```python
from build123d import *

# Parameters (mm, degrees)
BOSS_EXTRUDE7_DEPTH                          = 17
BOSS_EXTRUDE7_DEPTH_BACK                     = 17
SKETCH1_R                                    = 1.45
SKETCH34_W                                   = 28.4
SKETCH34_H                                   = 7.5
CUT_EXTRUDE11_DEPTH                          = 37.521397837
SKETCH35_R                                   = 5
CUT_EXTRUDE12_DEPTH                          = 25.542055741
CSK_FOR_M3_HEX_SOCKET_COUNTERSUNK_CA_2_COUNT = 2
CSK_FOR_M3_HEX_SOCKET_COUNTERSUNK_CA_2_PITCH = 16.5
CSK_FOR_M3_HEX_SOCKET_COUNTERSUNK_CA_3_COUNT = 2
CSK_FOR_M3_HEX_SOCKET_COUNTERSUNK_CA_3_PITCH = 18
CSK_FOR_M3_HEX_SOCKET_COUNTERSUNK_CA_4_COUNT = 2
CSK_FOR_M3_HEX_SOCKET_COUNTERSUNK_CA_4_PITCH = 24.418230894
FILLET5_R                                    = 1
SKETCH41_W                                   = 28.5
SKETCH41_H                                   = 0.4
CUT_EXTRUDE13_DEPTH                          = 40.895175147


with BuildPart() as part:
    # Sketch1 → Boss-Extrude7 (new, two sides: drawn at the far end of the back side and taken through both)
    # profile 1 of 3: a face of its own
    with BuildSketch(Plane.XY.offset(-BOSS_EXTRUDE7_DEPTH_BACK)):
        Polygon((-14.25, 15.25), (-14.25, 11.25), (-8.25, 11.25), (-8.25, 12.25), (8.25, 12.25), (8.25, 11.25), (14.25, 11.25), (14.25, 15.25), align=None)
    # profile 2 of 3: a face of its own
    with BuildSketch(Plane.XY.offset(-BOSS_EXTRUDE7_DEPTH_BACK)):
        with BuildLine():
            Line((14.25, 4.75), (14.25, 11.25))
            Line((14.25, 11.25), (8.25, 11.25))
            Line((8.25, 11.25), (8.25, 8.011710179))
            ThreePointArc((8.25, 8.011710179), (9.502581542, 6.476954843), (10.473180033, 4.75))
            Line((10.473180033, 4.75), (14.25, 4.75))
        make_face()
        with Locations((11, 8)):
            Circle(SKETCH1_R, mode=Mode.SUBTRACT)
    # profile 3 of 3: a face of its own
    with BuildSketch(Plane.XY.offset(-BOSS_EXTRUDE7_DEPTH_BACK)):
        with BuildLine():
            Line((-8.25, 11.25), (-14.25, 11.25))
            Line((-14.25, 11.25), (-14.25, 4.75))
            Line((-14.25, 4.75), (-10.473180033, 4.75))
            ThreePointArc((-10.473180033, 4.75), (-9.502581542, 6.476954843), (-8.25, 8.011710179))
            Line((-8.25, 8.011710179), (-8.25, 11.25))
        make_face()
        with Locations((-11, 8)):
            Circle(SKETCH1_R, mode=Mode.SUBTRACT)
    extrude(amount=BOSS_EXTRUDE7_DEPTH + BOSS_EXTRUDE7_DEPTH_BACK)

    # Sketch34 → Cut-Extrude11 (cut, through all)
    with BuildSketch(Plane.ZY.offset(14.25)):
        with Locations((0, 8.5)):
            Rectangle(SKETCH34_W, SKETCH34_H)
    extrude(amount=-CUT_EXTRUDE11_DEPTH, mode=Mode.SUBTRACT)

    # Sketch35 → Cut-Extrude12 (cut, through all)
    with BuildSketch(Plane(origin=(0, 15.25, 0), x_dir=(1, 0, 0), z_dir=(0, 1, 0))):
        with Locations(Location((0, 0, 0), (0, 0, 270))):
            Circle(SKETCH35_R)
    extrude(amount=-CUT_EXTRUDE12_DEPTH, mode=Mode.SUBTRACT)

    # Sketch40 → CSK for M3 Hex Socket Countersunk Cap Sc (revolve, cut)
    with BuildSketch(Plane(origin=(-8.25, 12.25, 9), x_dir=(0, 0, -1), z_dir=(1, 0, 0))):
        Polygon((0, 0), (0, 3), (1.7, 3), (1.7, 1.66), (3.36, 0), align=None)
    csk_for_m3_hex_socket_countersunk_cap_sc = revolve(axis=Axis((-8.25, 5.9, 9), (0, 1, 0)), mode=Mode.SUBTRACT)

    # CSK for M3 Hex Socket Countersunk Ca 2: CSK for M3 Hex Socket Countersunk Cap Sc ×2
    with Locations(*[(i * CSK_FOR_M3_HEX_SOCKET_COUNTERSUNK_CA_2_PITCH, 0, 0) for i in range(1, CSK_FOR_M3_HEX_SOCKET_COUNTERSUNK_CA_2_COUNT)]):
        add(csk_for_m3_hex_socket_countersunk_cap_sc, mode=Mode.SUBTRACT)

    # CSK for M3 Hex Socket Countersunk Ca 3: CSK for M3 Hex Socket Countersunk Cap Sc ×2
    with Locations(*[(0, 0, -i * CSK_FOR_M3_HEX_SOCKET_COUNTERSUNK_CA_3_PITCH) for i in range(1, CSK_FOR_M3_HEX_SOCKET_COUNTERSUNK_CA_3_COUNT)]):
        add(csk_for_m3_hex_socket_countersunk_cap_sc, mode=Mode.SUBTRACT)

    # CSK for M3 Hex Socket Countersunk Ca 4: CSK for M3 Hex Socket Countersunk Cap Sc ×2
    with Locations(*[Vector(0.6757246285173466, 0, -0.7371541402007413) * (i * CSK_FOR_M3_HEX_SOCKET_COUNTERSUNK_CA_4_PITCH) for i in range(1, CSK_FOR_M3_HEX_SOCKET_COUNTERSUNK_CA_4_COUNT)]):
        add(csk_for_m3_hex_socket_countersunk_cap_sc, mode=Mode.SUBTRACT)

    # Fillet5
    fillet5_edges = [part.edges().sort_by_distance(p)[0] for p in [
        (-14.25, 15.25, 0),
        (14.25, 15.25, 0),
        (0, 15.25, -17),
        (0, 15.25, 17),
    ]]
    fillet(fillet5_edges, radius=FILLET5_R)

    # Sketch41 → Cut-Extrude13 (cut, through all)
    with BuildSketch(Plane.XY.offset(17)):
        with Locations((0, 4.95)):
            Rectangle(SKETCH41_W, SKETCH41_H)
    extrude(amount=-CUT_EXTRUDE13_DEPTH, mode=Mode.SUBTRACT)


solid = part.part
```
Geometry check sheet. Reference: the model listing, model coordinates, mm. A direction names the side the tool comes from. Coordinates: 2 decimals unless noted, no trailing zeros. Order: outer loops, then holes, each group sorted by start corner. A loop starts at its lowest first (then second) coordinate and runs counter-clockwise, first axis right, second up. Notation, with made-up numbers: (11, 78) - (36, 78) arc R20 cw to (36, 92) - close; hole circle Ø1 at (1.25, -8). An arc over 180 degrees is marked (long way). Answer as a JSON object with one key per item and string values. Group by question number.
Item 1: Sectioned sample at A-A, the plane z = -9. Record the cut outline in (x, y), and give its area (3 significant figures).
Item 2: Depth check by flat-ended pin: pin 1 Ø1.8 at (x, y) = (-11.5, 9) entering from -Z. Enter the tip coordinate at first touch or a pass-through.
Item 3: Sectioned sample at B-B, the plane y = 10.5. Record the cut outline in (x, z).
Item 4: Sectioned sample at D-D, the plane x = -12. Record the cut outline in (y, z), and give its area (3 significant figures).
Item 5: Scan lines: probe 1 along X at (y, z) = (14.55, 9); probe 2 along Z at (x, y) = (12.25, 9.5); probe 3 along Z at (x, y) = (-8.25, 14.25). Record each from-to range of solid material in increasing order.
Item 6: Draft check along Y on faces 1 (the face through (8.2, 14.6, -7.3)), 2 (the face through (12, 5.15, 16)), 3 (the face through (9.85, 7.12, -15.62)). Enter one of: +Y half, -Y half, draft (parallel to the pull), parting line (faces both ways), or undercut.
Item 7: Sectioned sample at C-C, the plane z = 0. Record the cut outline in (x, y), and give its area (3 significant figures).
Item 8: Tool access check on faces 4 (the face through (9.36, 6.68, -15.62)), 5 (the face through (-12, 9.4, -14.2)), 6 (the face through (-12.15, 7.12, 15.58)). Record the directions out of +Z, -Z, +X, -X, +Y, -Y that give a thin tool (end or side, any length) a straight path to the whole face; none if there is none.
Resolved:
{
 "1": {"outline": "(-14.25, 12.25) - (-11.61, 12.25) - (-9.95, 13.91) - (-9.95, 15.25) - (-13.25, 15.25) arc R1 ccw to (-14.25, 14.25) - close; (-6.55, 13.91) - (-4.89, 12.25) - (4.89, 12.25) - (6.55, 13.91) - (6.55, 15.25) - (-6.55, 15.25) - close; (9.95, 13.91) - (11.61, 12.25) - (14.25, 12.25) - (14.25, 14.25) arc R1 ccw to (13.25, 15.25) - (9.95, 15.25) - close", "area": "59.2 mm^2"},
 "2": {"pin 1": "z = -17"},
 "3": {"outline": "(-14.25, -17) - (-8.25, -17) - (-8.25, -14.2) - (-14.25, -14.2) - close; (-14.25, 14.2) - (-8.25, 14.2) - (-8.25, 17) - (-14.25, 17) - close; (8.25, -17) - (14.25, -17) - (14.25, -14.2) - (8.25, -14.2) - close; (8.25, 14.2) - (14.25, 14.2) - (14.25, 17) - (8.25, 17) - close"},
 "4": {"outline": "(5.15, -17) - (6.95, -17) - (6.95, -14.2) - (5.15, -14.2) - close; (5.15, 14.2) - (6.95, 14.2) - (6.95, 17) - (5.15, 17) - close; (9.05, -17) - (14.25, -17) arc R1 ccw to (15.25, -16) - (15.25, 16) arc R1 ccw to (14.25, 17) - (9.05, 17) - (9.05, 14.2) - (12.25, 14.2) - (12.25, -14.2) - (9.05, -14.2) - close", "area": "130 mm^2"},
 "5": {"probe 1": "-14.2 to -9.95, -6.55 to 6.55, 9.95 to 14.2", "probe 2": "-17 to -14.2, 14.2 to 17", "probe 3": "-17 to -10.7, -7.3 to 7.3, 10.7 to 17"},
 "6": {"face 1": "draft", "face 2": "-Y half", "face 3": "undercut"},
 "7": {"outline": "(-14.25, 12.25) - (-5, 12.25) - (-5, 15.25) - (-13.25, 15.25) arc R1 ccw to (-14.25, 14.25) - close; (5, 12.25) - (14.25, 12.25) - (14.25, 14.25) arc R1 ccw to (13.25, 15.25) - (5, 15.25) - close", "area": "55.1 mm^2"},
 "8": {"face 4": "+Z, -Z, -Y", "face 5": "+X, -X, -Y", "face 6": "+Z, -Z"}
}
